Verification items for the finished model (mm, model axes). A direction names the side the tool comes from. Round coordinates to 2 decimals unless told otherwise and drop trailing zeros. Write each loop counter-clockwise with the first axis right and the second up, starting at its lowest first coordinate (ties: lowest second). Pieces come first, ordered by that corner, then holes. Notation, with made-up numbers: (-10, -39) - (28, -39) arc R30 cw to (28, 0) - close; hole circle Ø4 at (47, 1.5). An arc over 180 degrees is marked (long way). Answer as a JSON object with one key per item and string values. Group by question number.
1) Go/stop test with flat-tipped pins: pin 1 Ø1.3 at (x, y) = (1, -1) entering from -Z; pin 2 Ø1 at (y, z) = (-1.5, 3) entering from -X; pin 3 Ø1.5 at (x, z) = (1, 3.5) entering from +Y. Record where each tip stops, or that it passes through.
2) Section check A-A (y = 0). Enter the section's corners in (x, z).
3) Section check B-B (x = 0.6). Enter the section's corners in (y, z).
4) Set-up check for faces 4 (the flat face through (0, 0, 0)), 5 (the flat face through (0.49, 0.87, 8.06)): record each of +Z, -Z, +X, -X, +Y, -Y from which the full face is reachable in a straight line by a thin tool's end or side.
5) Section check C-C (z = 6.25). Enter the section's corners in (x, y), then the cut area to 3 significant figures.
6) Mould release check, pull along X, two halves, no side actions. Record for faces 1 (the flat face through (0, 0, 7.5)), 2 (the cylindrical face through (-0.17, -1.29, 2.96)), 3 (the flat face through (0, -1.5, 6)): +X half, -X half, draft (parallel to the pull), parting line (faces both ways), or undercut.
7) Thickness scan on line 1 (X direction, y = 0.6, z = 2.75); line 2 (Z direction, x = -0.65, y = 1.2). Record the ranges inside material, lowest first.
8) Section check D-D (z = 4.5). Enter the section's corners in (x, y), then the cut area to 3 significant figures.
Autodesk Inventor part; units mm, degrees
ref_plane "YZ Plane" through (0, 0, 0) normal (1, 0, 0) x (0, 1, 0)
ref_plane "XZ Plane" through (0, 0, 0) normal (0, 1, 0) x (-1, 0, 0)
ref_plane "XY Plane" through (0, 0, 0) normal (0, 0, 1) x (1, 0, 0)
sketch "スケッチ1" plane through (0, 0, 0) normal (0, 0, 1) x (1, 0, 0)
  circle A0 centre (0, 0) radius 1.3
  dimension "d0" = 2.6
extrude "押し出し1" add sketch "スケッチ1" along normal blind 6
sketch "スケッチ2" plane through (0, 0, 6) normal (0, 0, 1) x (1, 0, 0)
  circle A0 centre (0, 0) radius 1.3
  circle A1 centre (0, 0) radius 2.25
  dimension "d3" = 4.5
extrude "押し出し2" add sketch "スケッチ2" along normal blind 2.6 contours A0 | A1
sketch "スケッチ3" plane through (0, 0, 8.6) normal (0, 0, 1) x (1, 0, 0)
  circle A0 centre (0, 0) radius 2.25
  circle A1 centre (0, 0) radius 1.3
  line L0 (0, 1.1547) -> (1, 0.5774)
  line L1 (1, 0.5774) -> (1, -0.5774)
  line L2 (1, -0.5774) -> (0, -1.1547)
  line L3 (0, -1.1547) -> (-1, -0.5774)
  line L4 (-1, -0.5774) -> (-1, 0.5774)
  line L5 (-1, 0.5774) -> (0, 1.1547)
  dimension "d6" = 2
extrude "押し出し3" cut sketch "スケッチ3" against normal blind 1.1 contours L0 L1 L2 L3 L4 L5
thread "ねじ1"
properties part number "m2.6 6mm キャップボルト" material "鋼"
Returned:
{
 "1": {"pin 1": "z = 0", "pin 2": "x = -0.83", "pin 3": "y = 1.28"},
 "2": {"outline": "(-2.25, 6) - (-1.3, 6) - (-1.3, 0) - (1.3, 0) - (1.3, 6) - (2.25, 6) - (2.25, 8.6) - (1, 8.6) - (1, 7.5) - (-1, 7.5) - (-1, 8.6) - (-2.25, 8.6) - close"},
 "3": {"outline": "(-2.17, 6) - (-1.15, 6) - (-1.15, 0) - (1.15, 0) - (1.15, 6) - (2.17, 6) - (2.17, 8.6) - (0.81, 8.6) - (0.81, 7.5) - (-0.81, 7.5) - (-0.81, 8.6) - (-2.17, 8.6) - close"},
 "4": {"face 4": "-Z, +X, -X, +Y, -Y", "face 5": "+Z"},
 "5": {"outline": "circle Ø4.5 at (0, 0)", "area": "15.9 mm2"},
 "6": {"face 1": "undercut", "face 2": "parting line", "face 3": "draft"},
 "7": {"line 1": "-1.15 to 1.15", "line 2": "6 to 8.6"},
 "8": {"outline": "circle Ø2.6 at (0, 0)", "area": "5.31 mm2"}
}
